The figure shows three views and two pictorial views of one solid part (mm, origin at its lowest corner). Answer the questions. A direction names the side the tool comes from. Give positions to 0.01 mm unless a question says otherwise; leave off trailing zeros. Order: outer loops, then holes, each group sorted by start corner. A loop starts at its lowest first (then second) coordinate and runs counter-clockwise, first axis right, second up. Notation, with made-up numbers: (51.5, 41.25) - (94.5, 41.25) arc R26 cw to (94.5, 56.25) - close; hole circle Ø1 at (15.5, 33). An arc over 180 degrees is marked (long way). Write item = value, one per line.
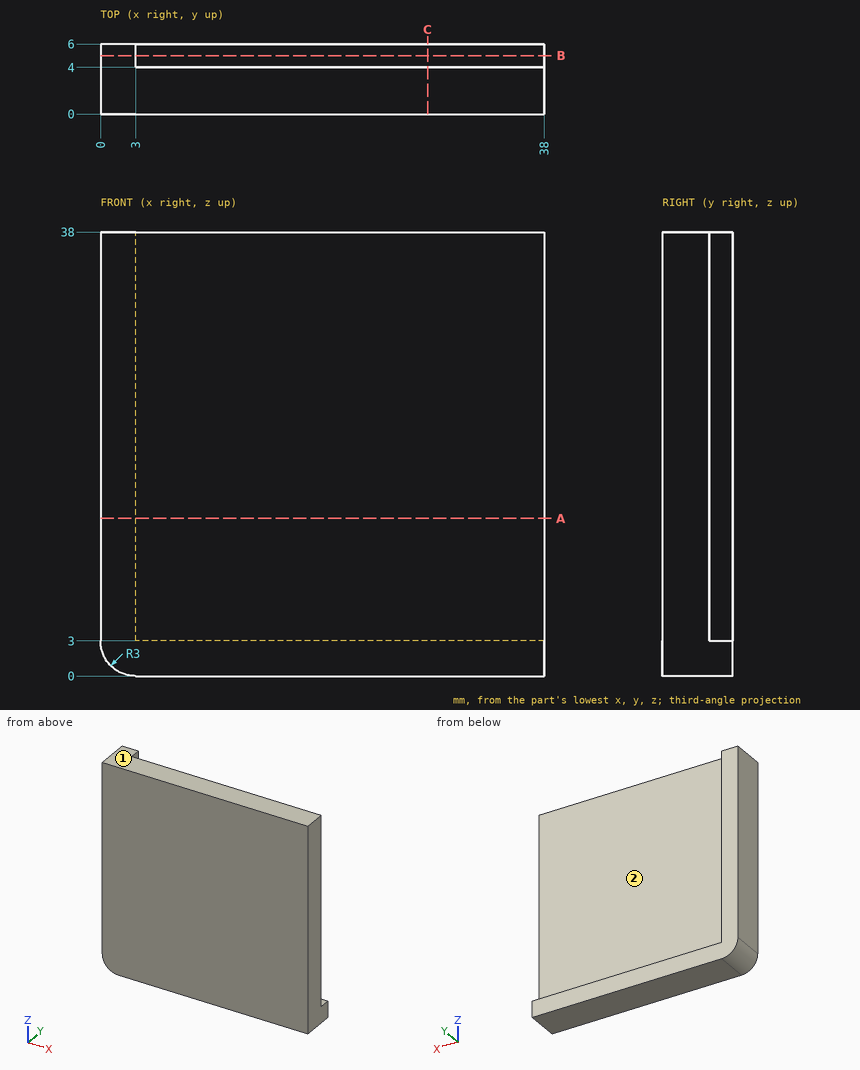
1. For the marked faces 1 and 2, determine the directions among +Z, -Z, +X, -X, +Y, -Y from which every point of the face is accessible in a straight line to the end or side of a thin tool.
Recorded:
face_1 = +Z, +X, -X, +Y, -Y
face_2 = +Z, +X, +Y
2. Section A-A (z = 13.5) is taken. Determine the outline of the cut face in (x, y).
Recorded:
outline = (0, 0) - (38, 0) - (38, 4) - (3, 4) - (3, 6) - (0, 6) - close
3. Section B-B (y = 5) is taken. Determine the outline of the cut face in (x, z).
Recorded:
outline = (0, 3) arc R3 ccw to (3, 0) - (38, 0) - (38, 3) - (3, 3) - (3, 38) - (0, 38) - close
4. Section C-C (x = 28) is taken. Determine the outline of the cut face in (y, z), and give its area (3 significant figures).
Recorded:
outline = (0, 0) - (6, 0) - (6, 3) - (4, 3) - (4, 38) - (0, 38) - close
area = 158 mm^2
5. Flat-ended cylindrical pins translate along their axes: pin 1 (10 mm diameter, centred on x = 21.5, z = 13, fed in from +Y); pin 2 (3 mm diameter, centred on x = 18, y = 1, fed in from -Z); pin 3 (0.6 mm diameter, centred on y = 4.5, z = 16, fed in from +X); pin 4 (0.6 mm diameter, centred on x = 28, y = 5, fed in from +Z). Find the tip coordinate at first contact, or state that the pin passes through.
Recorded:
pin_1 = 4
pin_2 = 0
pin_3 = 3
pin_4 = 3
6. Straight lines are drawn through the part: L1, parallel to Y at x = 12.5, z = 19; L2, parallel to Z at x = 31, y = 5.6. For each, find the intervals that lie inside material, in ascending order. Write a range as [from, to].
Recorded:
L1 = [0, 4]
L2 = [0, 3]
